For this review, take the finished solid that the model builds, in its own axes (mm). Face numbers are marked on the shaded views. A direction names the side the tool comes from. Coordinates: 2 decimals unless noted, no trailing zeros. Write each loop counter-clockwise with the first axis right and the second up, starting at its lowest first coordinate (ties: lowest second). Pieces come first, ordered by that corner, then holes. Notation, with made-up numbers: (-7, 18) - (48, 18) arc R32 ccw to (48, 47) - close; hole circle Ø7 at (42.5, -37.75). An arc over 180 degrees is marked (long way). Use one line per item in the form item = value. Start each with the question number.
1) We need section B-B (x = 18). Give the boundary of the cut face in (y, z), plus the area to 3 significant figures.
2) We need section A-A (z = 15.5). Give the boundary of the cut face in (x, y).
3) Mouldability with a two-part tool opening along X and no side actions: class the marked faces 3, 4, 5 and 6 as pulls with the +X half, pulls with the -X half, needs draft (parallel to the pull), parting line crosses it, or undercut.
4) Insertion check: P1, Ø20, axis at x = -6, z = 23.5, coming from the -Y side; P2, Ø2.5, axis at x = 28, z = 26.5, coming from the +Y side; P3, Ø10, axis at y = 33.5, z = 28, coming from the +X side; P4, Ø1.5, axis at y = 33.5, z = 60, coming from the +X side. Each pin has a flat end and moves straight along its axis. Give the tip position at first contact, or say it passes through.
5) Tool access review of the marked faces 1 and 2: name each direction out of +Z, -Z, +X, -X, +Y, -Y from which nothing blocks a thin tool from reaching the whole face with its end or side.
6) For L1, parallel to X at y = 14.25, z = 7.5; L2, parallel to Y at x = 11, z = 62.5; L3, parallel to Z at x = -4.5, y = 27, list the stretches that pass through material, from the lowest coordinate up. Write a range as from..to.
7) We need section C-C (z = 62.5). Give the boundary of the cut face in (x, y).
8) We need section D-D (y = 31.25). Give the boundary of the cut face in (x, z), plus the area to 3 significant figures.
```python
from build123d import *

# Parameters (mm, degrees)
F0_W     = 10
F0_H     = 1
F1_DEPTH = 70
F0_W_2   = 3
F0_H_2   = 9
F2_DEPTH = 40
F3_R     = 2
F4_R     = 3
F0_H_3   = 14
F5_DEPTH = 69
F6_SIZE2 = 10
F6_SIZE  = 30


with BuildPart() as f1:
    # F0 (on Top) → F1 (new body)
    with BuildSketch(Plane.XY):
        Polygon((33.5, 20.7614854574), (33.5, 23.7614854574), (32.5, 23.7614854574), (5, 23.7614854574), (5, 22.7614854574), (-5, 22.7614854574), (-5, 23.7614854574), (-33.5, 23.7614854574), (-33.5, 20.7614854574), (-30.5, 20.7614854574), (30.5, 20.7614854574), align=None)
        with Locations((0, 23.2614854574)):
            Rectangle(F0_W, F0_H)
    extrude(amount=F1_DEPTH)

    # F0 (on Top) → F2 (join)
    with BuildSketch(Plane.XY):
        Polygon((-25.5, 11.7614854574), (-30.5, 11.7614854574), (-33.5, 11.7614854574), (-33.5, 8.7614854574), (-25.5, 8.7614854574), align=None)
        with Locations((-32, 16.2614854574)):
            Rectangle(F0_W_2, F0_H_2)
        Polygon((33.5, 8.7614854574), (33.5, 11.7614854574), (30.5, 11.7614854574), (25.5, 11.7614854574), (25.5, 8.7614854574), align=None)
        with Locations((32, 16.2614854574)):
            Rectangle(F0_W_2, F0_H_2)
    extrude(amount=F2_DEPTH)

    # F3
    f3_edges = [f1.edges().sort_by_distance(p)[0] for p in [
        (33.5, 22.261485, 70),
        (-33.5, 22.261485, 70),
    ]]
    fillet(f3_edges, radius=F3_R)

    # F4
    f4_edges = [f1.edges().sort_by_distance(p)[0] for p in [
        (25.5, 10.261485, 40),
        (-25.5, 10.261485, 40),
    ]]
    fillet(f4_edges, radius=F4_R)

    # F0 (on Top) → F5 (join)
    with BuildSketch(Plane.XY):
        with Locations((0, 30.7614854574)):
            Rectangle(F0_W, F0_H_3)
    extrude(amount=F5_DEPTH)

    # F6
    f6_edges = [f1.edges().sort_by_distance(p)[0] for p in [
        (0, 37.761485, 69),
    ]]
    f6_side = f1.faces().sort_by_distance((0, 37.761485, 34.5))[0]
    chamfer(f6_edges, length=F6_SIZE, length2=F6_SIZE2, reference=f6_side)


solid = f1.part
```
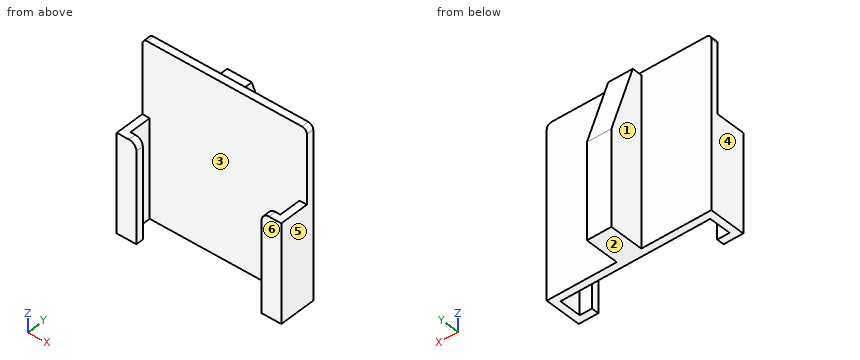
Determined:
q1.outline = (20.76, 0) - (23.76, 0) - (23.76, 70) - (20.76, 70) - close
q1.area = 210 mm²
q2.outline = (-33.5, 8.76) - (-25.5, 8.76) - (-25.5, 11.76) - (-30.5, 11.76) - (-30.5, 20.76) - (30.5, 20.76) - (30.5, 11.76) - (25.5, 11.76) - (25.5, 8.76) - (33.5, 8.76) - (33.5, 23.76) - (5, 23.76) - (5, 37.76) - (-5, 37.76) - (-5, 23.76) - (-33.5, 23.76) - close
q3.face_3 = undercut
q3.face_4 = pulls with the -X half
q3.face_5 = pulls with the +X half
q3.face_6 = needs draft
q4.P1 = 20.76
q4.P2 = 23.76
q4.P3 = 5
q4.P4 = through
q5.face_1 = +Z, -Z, -X, +Y
q5.face_2 = -Z, +X, -X, +Y, -Y
q6.L1 = -33.5..-30.5, 30.5..33.5
q6.L2 = 20.76..23.76
q6.L3 = 0..69
q7.outline = (-33.5, 20.76) - (33.5, 20.76) - (33.5, 23.76) - (5, 23.76) - (5, 29.93) - (-5, 29.93) - (-5, 23.76) - (-33.5, 23.76) - close
q8.outline = (-5, 0) - (5, 0) - (5, 58.53) - (-5, 58.53) - close
q8.area = 585 mm²
